Work out the finished part from the listing and answer in its coordinate system (mm). A direction names the side the tool comes from. Round coordinates to 2 decimals unless told otherwise and drop trailing zeros. Write each loop counter-clockwise with the first axis right and the second up, starting at its lowest first coordinate (ties: lowest second). Pieces come first, ordered by that corner, then holes. Notation, with made-up numbers: (47.5, 6.5) - (74.5, 6.5) arc R23 cw to (74.5, 22.5) - close; hole circle Ø2 at (79, -28.75). An arc over 180 degrees is marked (long way). Answer as a JSON object with one key per item and string values.
```python
from build123d import *

# Parameters (mm, degrees)
SKETCH_1_R             = 4
EXTRUDE_1_DEPTH        = 1.5
SKETCH_2_W             = 30
SKETCH_2_H             = 4
EXTRUDE_2_DEPTH        = 2
HOLE_WIZARD_M3_1_D     = 2.5
HOLE_WIZARD_M3_1_DEPTH = 2
HOLE_WIZARD_M3_1_TIP   = 0.751075774
CUT_EXTRUDE_2_DEPTH    = 10
HOLE_WIZARD_M2_1_D     = 1.6
HOLE_WIZARD_M2_1_DEPTH = 4.2
HOLE_WIZARD_M2_1_TIP   = 0.480688495


with BuildPart() as part:
    # 草图1 → 凸台-拉伸1 (new, symmetric)
    with BuildSketch(Plane.XY):
        with BuildLine():
            Line((11.33983382, 24), (6.893654271, -1.215537244))
            ThreePointArc((6.893654271, -1.215537244), (0, -7), (-6.893654271, -1.215537244))
            Line((-6.893654271, -1.215537244), (-11.33983382, 24))
            Line((-11.33983382, 24), (11.33983382, 24))
        make_face()
        Circle(SKETCH_1_R, mode=Mode.SUBTRACT)
    extrude(amount=EXTRUDE_1_DEPTH, both=True)

    # 草图2 → 凸台-拉伸2 (add)
    with BuildSketch(Plane(origin=(0, 24, 0), x_dir=(1, 0, 0), z_dir=(0, 1, 0))):
        Rectangle(SKETCH_2_W, SKETCH_2_H)
    extrude(amount=EXTRUDE_2_DEPTH)

    # M3 螺纹孔1
    with Locations(Plane(origin=(0, 26, 0), x_dir=(1, 0, 0), z_dir=(0, 1, 0))):
        with Locations((-13, 0), (13, 0)):
            Hole(HOLE_WIZARD_M3_1_D / 2, depth=HOLE_WIZARD_M3_1_DEPTH)
            with Locations((0, 0, -(HOLE_WIZARD_M3_1_DEPTH + HOLE_WIZARD_M3_1_TIP / 2))):  # 118° drill point
                Cone(0, HOLE_WIZARD_M3_1_D / 2, HOLE_WIZARD_M3_1_TIP, mode=Mode.SUBTRACT)

    # 草图8 → 切除-拉伸2 (cut)
    with BuildSketch(Plane(origin=(0, 0, -1.5), x_dir=(-1, 0, 0), z_dir=(0, 0, -1))):
        with BuildLine():
            Line((-1.5, 22), (-8.5, 22))
            Line((-8.5, 22), (-5.160522702, 3.060883114))
            ThreePointArc((-5.160522702, 3.060883114), (-3.602683726, 4.797986033), (-1.5, 5.809475019))
            Line((-1.5, 5.809475019), (-1.5, 22))
        make_face()
        with BuildLine():
            Line((8.5, 22), (1.5, 22))
            Line((1.5, 22), (1.5, 5.809475019))
            ThreePointArc((1.5, 5.809475019), (3.602683726, 4.797986033), (5.160522702, 3.060883114))
            Line((5.160522702, 3.060883114), (8.5, 22))
        make_face()
    extrude(amount=-CUT_EXTRUDE_2_DEPTH, mode=Mode.SUBTRACT)

    # M2 螺纹孔1
    with Locations(Plane(origin=(0, -7, 0), x_dir=(-1, 0, 0), z_dir=(0, -1, 0))):
        with Locations((0, 0)):
            Hole(HOLE_WIZARD_M2_1_D / 2, depth=HOLE_WIZARD_M2_1_DEPTH)
            with Locations((0, 0, -(HOLE_WIZARD_M2_1_DEPTH + HOLE_WIZARD_M2_1_TIP / 2))):  # 118° drill point
                Cone(0, HOLE_WIZARD_M2_1_D / 2, HOLE_WIZARD_M2_1_TIP, mode=Mode.SUBTRACT)


solid = part.part
```
Item 1: A cutting plane is placed at A-A (x = 13). Write down the section's boundary in (y, z), and give its area (3 significant figures).
Results found:
{"outline": "(24, -2) - (26, -2) - (26, -1.25) - (24, -1.25) - close; (24, 1.25) - (26, 1.25) - (26, 2) - (24, 2) - close", "area": "3.00 mm²"}
Item 2: Each of these flat-tipped pins is pushed along its axis until it touches: P1, Ø1, axis at y = 17, z = 1.5, coming from the +X side; P2, Ø1.5, axis at x = 3.5, z = -0.5, coming from the -Y side; P3, Ø18, axis at x = 3, y = 8.5, coming from the +Z side. Where does it stop, or does it pass through?
Results found:
{"P1": "x = 10.19", "P2": "y = -6.44", "P3": "z = 1.5"}
Item 3: A cutting plane is placed at B-B (y = 2). Write down the section's boundary in (x, z), and give its area (3 significant figures).
Results found:
{"outline": "(-7.46, -1.5) - (-3.46, -1.5) - (-3.46, 1.5) - (-7.46, 1.5) - close; (3.46, -1.5) - (7.46, -1.5) - (7.46, 1.5) - (3.46, 1.5) - close", "area": "24.0 mm²"}
Item 4: A cutting plane is placed at C-C (z = 0). Write down the section's boundary in (x, y).
Results found:
{"outline": "(-15, 24) - (-14.25, 24) - (-14.25, 26) - (-15, 26) - close; (-11.75, 24) - (-11.34, 24) - (-6.89, -1.22) arc R7 ccw to (-0.8, -6.95) - (-0.8, -3.92) arc R4 cw (long way) to (0.8, -3.92) - (0.8, -6.95) arc R7 ccw to (6.89, -1.22) - (11.34, 24) - (11.75, 24) - (11.75, 26) - (-11.75, 26) - close; (14.25, 24) - (15, 24) - (15, 26) - (14.25, 26) - close; hole (-8.5, 22) - (-5.16, 3.06) arc R6 cw to (-1.5, 5.81) - (-1.5, 22) - close; hole (1.5, 5.81) arc R6 cw to (5.16, 3.06) - (8.5, 22) - (1.5, 22) - close"}
Item 5: For faces 1 (the flat face through (6.854, 12.663, -0.021)), 2 (the flat face through (0, 12, 1.5)), 3 (the flat face through (-9.086, 11.216, 0.021)), 4 (the flat face through (-0.1, 24, 1.8)), 5 (the flat face through (0, 26, 0)), determine the directions among +Z, -Z, +X, -X, +Y, -Y from which every point of the face is accessible in a straight line to the end or side of a thin tool.
Results found:
{"face 1": "+Z, -Z", "face 2": "+Z, +X, -X, -Y", "face 3": "+Z, -Z, -X, -Y", "face 4": "-Y", "face 5": "+Z, -Z, +X, -X, +Y"}
Item 6: Consider line 1 along X through (y, z) = (11, -1.3); line 2 along Y through (x, z) = (-2, 0.8); line 3 along Z through (x, y) = (13, 25.05). Determine where each line is inside the solid, lowest interval first.
Results found:
{"line 1": "-9.05 to -6.56, -1.5 to 1.5, 6.56 to 9.05", "line 2": "-6.71 to -3.46, 3.46 to 5.66, 22 to 26", "line 3": "-2 to -1.25, 1.25 to 2"}
Item 7: A cutting plane is placed at D-D (x = -3.5). Write down the section's boundary in (y, z), and give its area (3 significant figures).
Results found:
{"outline": "(-6.06, -1.5) - (-1.94, -1.5) - (-1.94, 1.5) - (-6.06, 1.5) - close; (1.94, -1.5) - (4.87, -1.5) - (4.87, 1.5) - (1.94, 1.5) - close; (22, -1.5) - (24, -1.5) - (24, -2) - (26, -2) - (26, 2) - (24, 2) - (24, 1.5) - (22, 1.5) - close", "area": "35.2 mm²"}
Item 8: Determine the mould class of faces 6 (the flat face through (0, 25, 2)), 7 (the flat face through (-6.807, 12.398, -0.021)), 8 (the cylindrical face through (14.25, 24.99, -0.05)), 9 (the cylindrical face through (-0.63, -5.44, 0.49)) for opening direction Z: pulls with the +Z half, pulls with the -Z half, needs draft (parallel to the pull), parting line crosses it, or undercut.
Results found:
{"face 6": "pulls with the +Z half", "face 7": "needs draft", "face 8": "undercut", "face 9": "undercut"}
